Model file for the job. Use its own axes, mm. Face numbers are marked on the shaded views. A direction names the side the tool comes from. Coordinates: 2 decimals unless noted, no trailing zeros. Write each loop counter-clockwise with the first axis right and the second up, starting at its lowest first coordinate (ties: lowest second). Pieces come first, ordered by that corner, then holes. Notation, with made-up numbers: M 43,1.25 L 84,1.25 A27 cw 84,25.25 Z; hole C 30.5,88 d1. An arc over 180 degrees is marked long. Put each result on its own line as item: value. Start each with the question number.
Q1. Which spindle directions (+Z, -Z, +X, -X, +Y, -Y) get a long thin tool onto all of the face, cutting with end or side? Do the marked faces 1, 2, 3 and 4. Say none if no direction does.
Q2. Cut at A-A (z = 0.05). Write the cut outline in (x, y).
Q3. Drop flat-ended pins along their axis: pin 1 (1 mm diameter, centred on x = 1.5, y = 5.5, fed in from -Z); pin 2 (0.5 mm diameter, centred on x = -3.5, z = 0, fed in from -Y); pin 3 (0.8 mm diameter, centred on y = 8, z = 0, fed in from -X); pin 4 (1.1 mm diameter, centred on y = 9.5, z = 0, fed in from +X). Give the stop position or say it passes through.
Q4. Drill centre lines: line 1 along Y through (x, z) = (0, 0.3); line 2 along X through (y, z) = (16, -0.05); line 3 along Y through (x, z) = (1.25, -0.05). Where is each one in solid material? Low to high.
Q5. Cut at B-B (x = 7). Write the cut outline in (y, z).
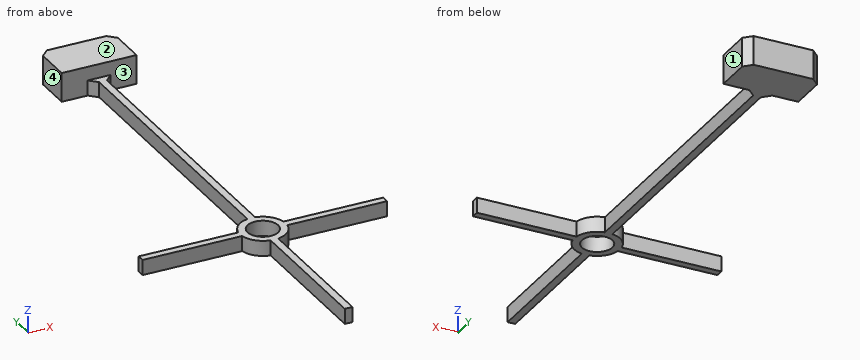
```python
from build123d import *

# Parameters (mm, degrees)
SKETCH_1_R          = 1
EXTRUDE_1_DEPTH     = 0.5
SKETCH_2_W          = 4.9
SKETCH_2_H          = 2.9
EXTRUDE_2_DEPTH     = 1.4
SKETCH_2_2_W        = 4.9
SKETCH_2_2_H        = 2.9
EXTRUDE_3_DEPTH     = 0.5
CHAMFER_1_SIZE      = 0.5
CHAMFER_2_SIZE      = 0.5
SKETCH_3_W          = 11.619186974
SKETCH_3_H          = 20
CUT_EXTRUDE_1_DEPTH = 5


with BuildPart() as part:
    # 스케치1 → 보스-돌출1 (new, symmetric)
    with BuildSketch(Plane.XY):
        with BuildLine():
            ThreePointArc((-0.25, -1.479019946), (-1.060660172, -1.060660172), (-1.479019946, -0.25))
            Line((-1.479019946, -0.25), (-8, -0.25))
            Line((-8, -0.25), (-8, 0.25))
            Line((-8, 0.25), (-1.479019946, 0.25))
            ThreePointArc((-1.479019946, 0.25), (-1.060660172, 1.060660172), (-0.25, 1.479019946))
            Line((-0.25, 1.479019946), (-0.25, 21))
            Line((-0.25, 21), (0.25, 21))
            Line((0.25, 21), (0.25, 1.479019946))
            ThreePointArc((0.25, 1.479019946), (1.060660172, 1.060660172), (1.479019946, 0.25))
            Line((1.479019946, 0.25), (8, 0.25))
            Line((8, 0.25), (8, -0.25))
            Line((8, -0.25), (1.479019946, -0.25))
            ThreePointArc((1.479019946, -0.25), (1.060660172, -1.060660172), (0.25, -1.479019946))
            Line((0.25, -1.479019946), (0.25, -21))
            Line((0.25, -21), (-0.25, -21))
            Line((-0.25, -21), (-0.25, -1.479019946))
        make_face()
        Circle(SKETCH_1_R, mode=Mode.SUBTRACT)
    extrude(amount=EXTRUDE_1_DEPTH, both=True)

    # 스케치2 → 보스-돌출2 (add)
    with BuildSketch(Plane.XY):
        with Locations((0, 22.45)):
            Rectangle(SKETCH_2_W, SKETCH_2_H)
    extrude(amount=EXTRUDE_2_DEPTH)

    # 스케치2<2> → 보스-돌출3 (add)
    with BuildSketch(Plane.XY):
        with Locations((0, 22.45)):
            Rectangle(SKETCH_2_2_W, SKETCH_2_2_H)
    extrude(amount=-EXTRUDE_3_DEPTH)

    # 모따기1
    chamfer_1_edges = [part.edges().sort_by_distance(p)[0] for p in [
        (2.45, 23.9, 0.45),
        (-2.45, 23.9, 0.45),
    ]]
    chamfer(chamfer_1_edges, length=CHAMFER_1_SIZE)

    # 모따기2
    chamfer_2_edges = [part.edges().sort_by_distance(p)[0] for p in [
        (-0.25, 21, 0),
        (0.25, 21, 0),
    ]]
    chamfer(chamfer_2_edges, length=CHAMFER_2_SIZE)

    # 스케치3 → 컷-돌출1 (cut, symmetric)
    with BuildSketch(Plane.XY):
        with Locations((0, -21)):
            Rectangle(SKETCH_3_W, SKETCH_3_H)
    extrude(amount=CUT_EXTRUDE_1_DEPTH, both=True, mode=Mode.SUBTRACT)


solid = part.part
```
Computed values:
1. face 1: +Z, -Z, +X, +Y
1. face 2: +Z, +X, -X, +Y, -Y
1. face 3: +Z
1. face 4: +Z, -Z, -X, +Y
2. outline: M -8,-0.25 L -1.48,-0.25 A1.5 ccw -0.25,-1.48 L -0.25,-11 L 0.25,-11 L 0.25,-1.48 A1.5 ccw 1.48,-0.25 L 8,-0.25 L 8,0.25 L 1.48,0.25 A1.5 ccw 0.25,1.48 L 0.25,20.5 L 0.75,21 L 2.45,21 L 2.45,23.4 L 1.95,23.9 L -1.95,23.9 L -2.45,23.4 L -2.45,21 L -0.75,21 L -0.25,20.5 L -0.25,1.48 A1.5 ccw -1.48,0.25 L -8,0.25 Z; hole C 0,0 d2
3. pin 1: through
3. pin 2: y = -0.25
3. pin 3: x = -0.25
3. pin 4: x = 0.25
4. line 1: -11 to -1, 1 to 23.9
4. line 2: -0.25 to 0.25
4. line 3: -0.83 to 0.83, 21 to 23.9
5. outline: M -0.25,-0.5 L 0.25,-0.5 L 0.25,0.5 L -0.25,0.5 Z
